Model file for the job. Use its own axes, mm. Face numbers are marked on the shaded views. Coordinates: 2 decimals unless noted, no trailing zeros. Write each loop counter-clockwise with the first axis right and the second up, starting at its lowest first coordinate (ties: lowest second). Pieces come first, ordered by that corner, then holes. Notation, with made-up numbers: (89, 71.25) -> (106, 71.25) arc R23 cw to (106, 101.25) -> close; hole circle Ø1 at (48.5, -38). An arc over 180 degrees is marked (long way). Write item = value, one per line. Start each with the question number.
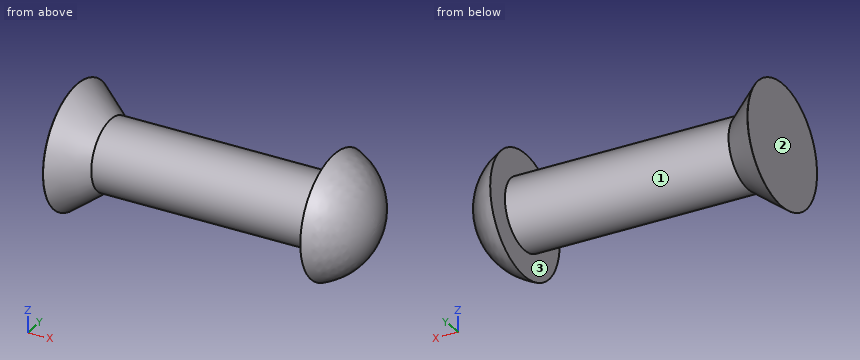
Autodesk Inventor part; units mm, degrees
ref_plane "YZ Plane" through (0, 0, 0) normal (1, 0, 0) x (0, 1, 0)
ref_plane "XZ Plane" through (0, 0, 0) normal (0, 1, 0) x (-1, 0, 0)
ref_plane "XY Plane" through (0, 0, 0) normal (0, 0, 1) x (1, 0, 0)
sketch "Sketch" plane through (0, 0, 0) normal (0, 0, 1) x (1, 0, 0)
  line L0 (0, 0) -> (0, 2.6)
  line L1 (0, 2.6) -> (0.0065, 2.6)
  line L2 (0.0065, 2.6) -> (1.44, 1.5)
  line L3 (1.44, 1.5) -> (11.001, 1.5)
  line L4 (11.001, 1.5) -> (11.001, 2.6)
  line L5 (0, 0) -> (12.801, 0)
  arc A0 (12.801, 0) -> (11.001, 2.6) centre (10.0232, 0) ccw
  line L6 (-0.2879, 0) -> (1.7274, 0)
  line L7 (0, -0.2166) -> (0, 1.2997)
  dimension "d0" = 5.2
  dimension "d1" = 3
  dimension "d2" = 5.2
  dimension "d3" = 1.44
  dimension "d4" = 1.8
  dimension "d5" = 11.001
  dimension "d6" = 37.5
revolve "Body" add sketch "Sketch" angle 360 about axis through (0, 0, 0) along (1, 0, 0)
equation "\"d0\" = KOD"
equation "\"d1\" = NND1"
equation "\"d2\" = KOD1"
equation "\"d3\" = KOH"
equation "\"d4\" = KOH1"
equation "\"d6\" = 0.5 * SEWI"
equation "\"KLG\" = 11"
equation "\"NND1\" = 3"
equation "\"KOH\" = 1.44"
equation "\"KOD\" = 5.2"
equation "\"SEWI\" = 75deg"
equation "\"KOH1\" = 1.8"
equation "\"KOD1\" = 5.2"
equation "\"NLG\" = 16"
equation "\"KLGMIN\" = 1.8"
equation "\"NND\" = 3"
equation "\"KLGMAX\" = 11"
properties part number "DIN 661 - A 3 x 16" material "Steel, Mild"
(1) Saw through at A-A (x = 7.25). Give the cut face in (y, z).
(2) Mould opens along X. For the marked faces 1, 2 and 3 say: released by +X, released by -X, zero draft, split by the parting line, or undercut.
(3) Drop flat-ended pins along their axis: pin 1 Ø2 at (x, y) = (3, -1) entering from -Z; pin 2 Ø1 at (y, z) = (-2, 0.5) entering from +X. Give the stop position or say it passes through.
(4) Drill centre lines: line 1 along Y through (x, z) = (6.25, 0.05); line 2 along X through (y, z) = (0.95, -1.2); line 3 along X through (y, z) = (0.8, -2.25). Where is each one in solid material? Low to high.
Returned:
q1.outline = circle Ø3 at (0, 0)
q2.face_1 = undercut
q2.face_2 = released by -X
q2.face_3 = undercut
q3.pin_1 = -1.5
q3.pin_2 = 12.32
q4.line_1 = -1.5 to 1.5
q4.line_2 = 0 to 1.4, 11 to 12.34
q4.line_3 = 0 to 0.28, 11 to 11.44
